For this review, use the dimensioned drawing (mm, ordinates from the lowest corner) and the shaded views. A direction names the side the tool comes from. Coordinates: 2 decimals unless noted, no trailing zeros. Write each loop counter-clockwise with the first axis right and the second up, starting at its lowest first coordinate (ties: lowest second). Pieces come first, ordered by that corner, then holes. Notation, with made-up numbers: M 32,22 L 57,22 A22 ccw 57,45 Z; hole C 77.5,19.25 d5. An arc over 180 degrees is marked long. Return JSON: item names as keys, results as strings. Group by question number.
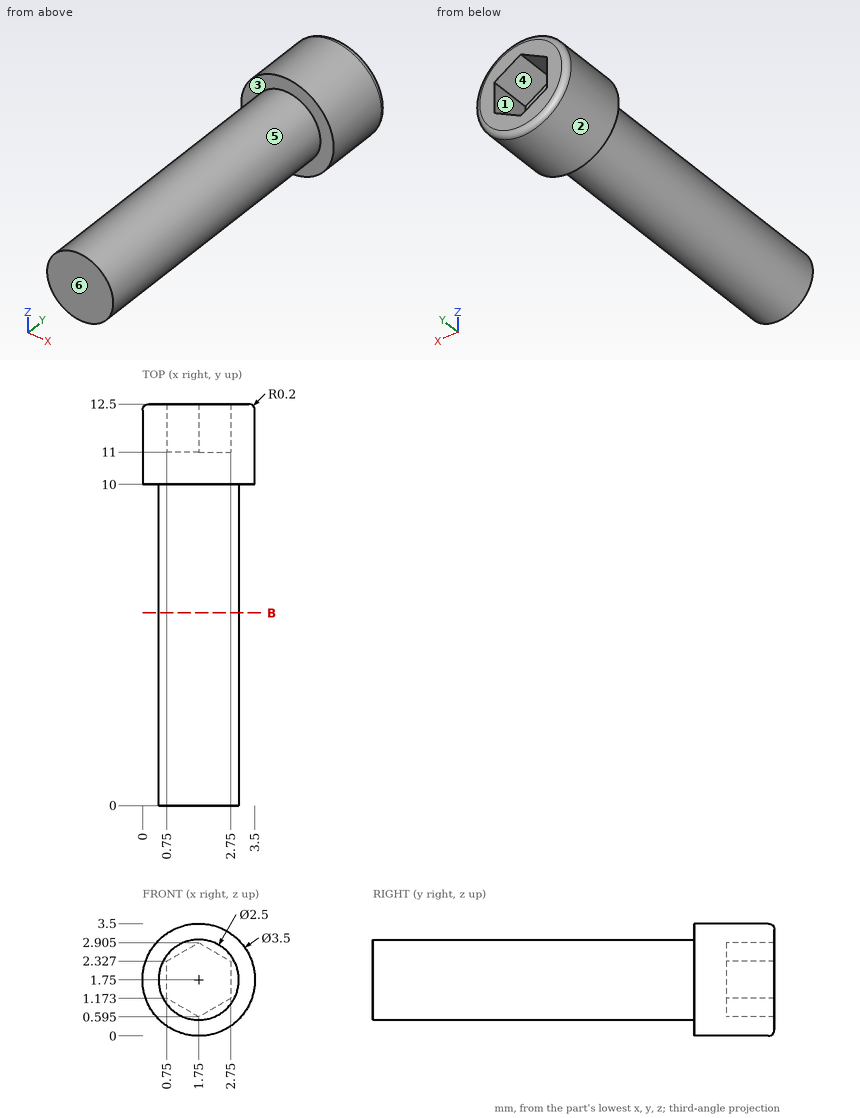
Item 1: Add section B-B (y = 6). Write out the cut boundary in (x, z).
Item 2: The part is to be moulded in two halves that separate along X. For the marked faces 1, 2 and 3, say which applies: pulls with the +X half, pulls with the -X half, needs draft (parallel to the pull), parting line crosses it, or undercut.
Item 3: For pin 1 (1 mm diameter, centred on x = 1, z = 1, fed in from -Y); pin 2 (1.5 mm diameter, centred on y = 2, z = 3, fed in from -X) (1 decimal), all flat-tipped, find the tip position at first contact; note any pin that passes through.
Item 4: Machinability: for the marked faces 4, 5 and 6, which of the approach directions +Z, -Z, +X, -X, +Y, -Y give a long, thin tool a straight path to every point of the face, cutting with its end or side? Answer none if there is none.
Item 5: For line 1 (Y direction, x = 1.05, z = 1.2); line 2 (Y direction, x = 0.4, z = 2.55); line 3 (X direction, y = 11.25, z = 1.3), list the stretches that pass through material, from the lowest coordinate up.
Geometry check:
{
 "1": {"outline": "C 1.75,1.75 d2.5"},
 "2": {"face 1": "undercut", "face 2": "parting line crosses it", "face 3": "needs draft"},
 "3": {"pin 1": "y = 0", "pin 2": "x = 0.6"},
 "4": {"face 4": "+Y", "face 5": "-Y", "face 6": "+Z, -Z, +X, -X, -Y"},
 "5": {"line 1": "0 to 11", "line 2": "10 to 12.5", "line 3": "0.06 to 0.75, 2.75 to 3.44"}
}
